Model file for the job. Use its own axes, mm. A direction names the side the tool comes from. Coordinates: 2 decimals unless noted, no trailing zeros. Write each question's results on one line, items separated by ' | '. Start each with the question number.
```python
from build123d import *

# Parameters (mm, degrees)
SKETCH1_R           = 2.1
BOSS_EXTRUDE1_DEPTH = 310


with BuildPart() as part:
    # Sketch1 → Boss-Extrude1 (new body)
    with BuildSketch(Plane(origin=(0, 0, 0), x_dir=(0, 0, -1), z_dir=(1, 0, 0))):
        with BuildLine():
            Line((-10, 9), (-10, 3))
            Line((-10, 3), (-8, 3))
            Line((-8, 3), (-8, 6))
            Line((-8, 6), (-7.060660172, 6))
            Line((-7.060660172, 6), (-4, 2.939339828))
            Line((-4, 2.939339828), (-4, -2.939339828))
            Line((-4, -2.939339828), (-7.060660172, -6))
            Line((-7.060660172, -6), (-8, -6))
            Line((-8, -6), (-8, -3))
            Line((-8, -3), (-10, -3))
            Line((-10, -3), (-10, -9))
            ThreePointArc((-10, -9), (-9.707106781, -9.707106781), (-9, -10))
            Line((-9, -10), (-3, -10))
            Line((-3, -10), (-3, -8))
            Line((-3, -8), (-6, -8))
            Line((-6, -8), (-6, -7.060660172))
            Line((-6, -7.060660172), (-2.939339828, -4))
            Line((-2.939339828, -4), (2.939339828, -4))
            Line((2.939339828, -4), (6, -7.060660172))
            Line((6, -7.060660172), (6, -8))
            Line((6, -8), (3, -8))
            Line((3, -8), (3, -10))
            Line((3, -10), (9, -10))
            ThreePointArc((9, -10), (9.707106781, -9.707106781), (10, -9))
            Line((10, -9), (10, -3))
            Line((10, -3), (8, -3))
            Line((8, -3), (8, -6))
            Line((8, -6), (7.060660172, -6))
            Line((7.060660172, -6), (4, -2.939339828))
            Line((4, -2.939339828), (4, 2.939339828))
            Line((4, 2.939339828), (7.060660172, 6))
            Line((7.060660172, 6), (8, 6))
            Line((8, 6), (8, 3))
            Line((8, 3), (10, 3))
            Line((10, 3), (10, 9))
            ThreePointArc((10, 9), (9.707106781, 9.707106781), (9, 10))
            Line((9, 10), (3, 10))
            Line((3, 10), (3, 8))
            Line((3, 8), (6, 8))
            Line((6, 8), (6, 7.060660172))
            Line((6, 7.060660172), (2.939339828, 4))
            Line((2.939339828, 4), (-2.939339828, 4))
            Line((-2.939339828, 4), (-6, 7.060660172))
            Line((-6, 7.060660172), (-6, 8))
            Line((-6, 8), (-3, 8))
            Line((-3, 8), (-3, 10))
            Line((-3, 10), (-9, 10))
            ThreePointArc((-9, 10), (-9.707106781, 9.707106781), (-10, 9))
        make_face()
        Circle(SKETCH1_R, mode=Mode.SUBTRACT)
    extrude(amount=BOSS_EXTRUDE1_DEPTH)


solid = part.part
```
Q1. Drill centre lines: L1, parallel to Y at x = 51.5, z = 8.25; L2, parallel to Z at x = 178, y = -7.5; L3, parallel to Y at x = 33, z = -0.5. Where is each one in solid material? Low to high. Write a range as from..to.
Q2. Which spindle directions (+Z, -Z, +X, -X, +Y, -Y) get a long thin tool onto all of the face, cutting with end or side? Do faces 5 (the flat face through (153, 0, 4)), 6 (the flat face through (153, -6, 10)), 7 (the flat face through (153, 0, -4)). Say none if no direction does.
Q3. Mould opens along Z. For faces 1 (the flat face through (153, 6, -10)), 2 (the flat face through (153, 4, 0)), 3 (the flat face through (310, 2.4, 0.1)), 4 (the flat face through (153, -4, 0)) say: +Z half, -Z half, draft (parallel to the pull), parting line (faces both ways), or undercut.
Q4. Pin check, flat tips, straight feed: pin 1 (10 mm diameter, centred on y = -7, z = -6, fed in from -X); pin 2 (1.8 mm diameter, centred on x = 132, z = -1.5, fed in from +Y); pin 3 (3 mm diameter, centred on x = 178.5, y = -1, fed in from +Z); pin 4 (4.5 mm diameter, centred on x = 113.5, y = 0.5, fed in from -Z). Stop position of each tip, or through.
Check result:
1) L1: -10..-3, 3..10 | L2: -10..-6, 6..10 | L3: -4..-2.04, 2.04..4
2) face 5: +Z, +X, -X | face 6: +Z, +X, -X, +Y, -Y | face 7: -Z, +X, -X
3) face 1: -Z half | face 2: undercut | face 3: draft | face 4: undercut
4) pin 1: x = 0 | pin 2: y = 4 | pin 3: z = 4 | pin 4: z = -4
